```python
from build123d import *

# Parameters (mm, degrees)
SKETCH1_W           = 15
SKETCH1_H           = 18
BOSS_EXTRUDE1_DEPTH = 6
SKETCH2_W           = 11
SKETCH2_H           = 11
CUT_EXTRUDE1_DEPTH  = 4
SKETCH3_W           = 4
SKETCH3_H           = 5
BOSS_EXTRUDE2_DEPTH = 11


with BuildPart() as part:
    # Sketch1 → Boss-Extrude1 (new body)
    with BuildSketch(Plane.XY):
        with Locations((7.5, 9)):
            Rectangle(SKETCH1_W, SKETCH1_H)
    extrude(amount=BOSS_EXTRUDE1_DEPTH)

    # Sketch2 → Cut-Extrude1 (cut)
    with BuildSketch(Plane.XY.offset(6)):
        with Locations((7.5, 9)):
            Rectangle(SKETCH2_W, SKETCH2_H)
    extrude(amount=-CUT_EXTRUDE1_DEPTH, mode=Mode.SUBTRACT)

    # Sketch3 → Boss-Extrude2 (add)
    with BuildSketch(Plane(origin=(0, 0, 0), x_dir=(-1, 0, 0), z_dir=(0, 0, -1))):
        with Locations((-12, 14)):
            Rectangle(SKETCH3_W, SKETCH3_H)
        with Locations((-3, 14)):
            Rectangle(SKETCH3_W, SKETCH3_H)
        with Locations((-12, 4)):
            Rectangle(SKETCH3_W, SKETCH3_H)
        with Locations((-3, 4)):
            Rectangle(SKETCH3_W, SKETCH3_H)
    extrude(amount=BOSS_EXTRUDE2_DEPTH)


solid = part.part
```
Check sheet for the modelled part. Datum: model origin and axes. Units: mm. A direction names the side the tool comes from. Coordinates: 2 decimals unless noted, no trailing zeros. Loops run counter-clockwise (first coordinate to the right, second up) from the corner with the lowest first, then second, coordinate; pieces in that order, holes last. Notation, with made-up numbers: M 27,23 L 70,23 A15 ccw 70,50 Z; hole C -30,85 d8. An arc over 180 degrees is marked long. Answer as a JSON object with one key per item and string values.
1. Scan lines: L1, parallel to Y at x = 10, z = 2.25; L2, parallel to X at y = 13, z = -6; L3, parallel to Y at x = 11.25, z = -5. Record each from-to range of solid material in increasing order. Write a range as from..to.
Outcome:
{"L1": "0..3.5, 14.5..18", "L2": "1..5, 10..14", "L3": "1.5..6.5, 11.5..16.5"}
2. Release check for a two-part mould opening along X. For faces 4 (the flat face through (5, 4, -5)), 5 (the flat face through (10, 14, -5)), 6 (the flat face through (3, 1.5, -5)), 7 (the flat face through (0, 9, 3)) record: pulls with the +X half, pulls with the -X half, needs draft (parallel to the pull), parting line crosses it, or undercut.
Outcome:
{"face 4": "undercut", "face 5": "undercut", "face 6": "needs draft", "face 7": "pulls with the -X half"}
3. Sectioned sample at D-D on z = 5.25. Record the cut outline in (x, y), and give its area (3 significant figures).
Outcome:
{"outline": "M 0,0 L 15,0 L 15,18 L 0,18 Z; hole M 2,3.5 L 13,3.5 L 13,14.5 L 2,14.5 Z", "area": "149 mm²"}
4. Sectioned sample at C-C on y = 3.75. Record the cut outline in (x, z).
Outcome:
{"outline": "M 0,0 L 1,0 L 1,-11 L 5,-11 L 5,0 L 10,0 L 10,-11 L 14,-11 L 14,0 L 15,0 L 15,6 L 13,6 L 13,2 L 2,2 L 2,6 L 0,6 Z"}
5. Access from +Z, -Z, +X, -X, +Y, -Y to the whole of each face (thin tool, end or side, straight path). Record for faces 1 (the flat face through (12, 16.5, -5)), 2 (the flat face through (7, 3.5, 4)), 3 (the flat face through (5, 14, -5)).
Outcome:
{"face 1": "-Z, +X, -X, +Y", "face 2": "+Z", "face 3": "-Z, +Y, -Y"}
6. Sectioned sample at A-A on z = -5.5. Record the cut outline in (x, y), and give its area (3 significant figures).
Outcome:
{"outline": "M 1,1.5 L 5,1.5 L 5,6.5 L 1,6.5 Z; M 1,11.5 L 5,11.5 L 5,16.5 L 1,16.5 Z; M 10,1.5 L 14,1.5 L 14,6.5 L 10,6.5 Z; M 10,11.5 L 14,11.5 L 14,16.5 L 10,16.5 Z", "area": "80.0 mm²"}
7. Sectioned sample at B-B on x = 2.5. Record the cut outline in (y, z), and give its area (3 significant figures).
Outcome:
{"outline": "M 0,0 L 1.5,0 L 1.5,-11 L 6.5,-11 L 6.5,0 L 11.5,0 L 11.5,-11 L 16.5,-11 L 16.5,0 L 18,0 L 18,6 L 14.5,6 L 14.5,2 L 3.5,2 L 3.5,6 L 0,6 Z", "area": "174 mm²"}
8. Depth check by flat-ended pin: P1, Ø1.5, axis at y = 15, z = -6.5, coming from the +X side; P2, Ø2, axis at x = 4.5, y = 7.5, coming from the +Z side; P3, Ø3, axis at x = 11, z = -3.5, coming from the -Y side. Enter the tip coordinate at first touch or a pass-through.
Outcome:
{"P1": "x = 14", "P2": "z = 2", "P3": "y = 1.5"}
